Design review of the part built by this model. Coordinates are the model's own, in mm. Coordinates: 2 decimals unless noted, no trailing zeros. Write each loop counter-clockwise with the first axis right and the second up, starting at its lowest first coordinate (ties: lowest second). Pieces come first, ordered by that corner, then holes. Notation, with made-up numbers: M 32.5,-36.5 L 77.5,-36.5 A35 cw 77.5,-3.5 Z; hole C -2.75,62.5 d9. An arc over 180 degrees is marked long. Write item = value, one per line.
```python
from build123d import *

# Parameters (mm, degrees)
BOSS_EXTRUDE2_DEPTH     = 1.5875
SKETCH2_W               = 38.1
SKETCH2_H               = 76.2
BOSS_EXTRUDE3_DEPTH     = 4.7625
CUT_EXTRUDE1_DEPTH      = 1.5875
CHAMFER1_SIZE           = 2
CUT_EXTRUDE2_DEPTH      = 306.117964892
CUT_EXTRUDE2_DEPTH_BACK = 306.117964892
SKETCH4_R               = 1.25


with BuildPart() as part:
    # Sketch1 → Boss-Extrude2 (new, symmetric)
    with BuildSketch(Plane.XY.offset(250.46101)):
        with BuildLine():
            Line((-62.9, 238.2), (-40.1, 238.2))
            ThreePointArc((-40.1, 238.2), (-30.200505063, 234.099494937), (-26.1, 224.2))
            Line((-26.1, 224.2), (-26.1, -219))
            Line((-26.1, -219), (-26.1, -295.2))
            Line((-26.1, -295.2), (-76.9, -295.2))
            Line((-76.9, -295.2), (-76.9, -219))
            Line((-76.9, -219), (-76.9, 224.2))
            ThreePointArc((-76.9, 224.2), (-72.799494937, 234.099494937), (-62.9, 238.2))
        make_face()
    extrude(amount=BOSS_EXTRUDE2_DEPTH, both=True)

    # Sketch2 → Boss-Extrude3 (add, symmetric)
    with BuildSketch(Plane.XY.offset(250.46101)):
        with Locations((-51.5, -257.1)):
            Rectangle(SKETCH2_W, SKETCH2_H)
        with BuildLine():
            Line((-60.39, 231.85), (-42.61, 231.85))
            ThreePointArc((-42.61, 231.85), (-35.425795103, 228.874204897), (-32.45, 221.69))
            Line((-32.45, 221.69), (-32.45, -219))
            Line((-32.45, -219), (-70.55, -219))
            Line((-70.55, -219), (-70.55, 221.69))
            ThreePointArc((-70.55, 221.69), (-67.574204897, 228.874204897), (-60.39, 231.85))
        make_face()
    extrude(amount=BOSS_EXTRUDE3_DEPTH, both=True)

    # Sketch3 → Cut-Extrude1 (cut)
    with BuildSketch(Plane.XY.offset(255.22351)):
        with BuildLine():
            Line((-61.025, -95.175), (-61.025, -213.725))
            Line((-61.025, -213.725), (-41.975, -213.725))
            Line((-41.975, -213.725), (-41.975, -95.175))
            ThreePointArc((-41.975, -95.175), (-42.90493597, -92.92993597), (-45.15, -92))
            Line((-45.15, -92), (-57.85, -92))
            ThreePointArc((-57.85, -92), (-60.09506403, -92.92993597), (-61.025, -95.175))
        make_face()
    cut_extrude1 = extrude(amount=-CUT_EXTRUDE1_DEPTH, mode=Mode.SUBTRACT)

    # Mirror2: Cut-Extrude1 across plane
    add(cut_extrude1.mirror(Plane.XY.offset(250.46101)), mode=Mode.SUBTRACT)

    # Chamfer1
    # the kernel refuses this chamfer: 2 mm, written as the material it takes off along each edge
    with BuildSketch(Plane(origin=(-41.975, -213.725, 255.22351), x_dir=(0.999621916911297, 0, 0.0274958766105822), z_dir=(0, 1, 0))) as chamfer1_piece_1_section:
        Polygon((CHAMFER1_SIZE * 0.999621916911, CHAMFER1_SIZE * 0.0274958766106), (-CHAMFER1_SIZE * 0.0274958766106, CHAMFER1_SIZE * 0.999621916911), (0, 0), align=None)
    chamfer1_piece_1 = extrude(amount=118.55, mode=Mode.PRIVATE)
    chamfer1_piece_1 = split(chamfer1_piece_1, bisect_by=Plane(origin=(-41.282092609, -154.45, 253.63601), z_dir=(0, 0, 1)), keep=Keep.TOP, mode=Mode.PRIVATE)
    add(chamfer1_piece_1, mode=Mode.SUBTRACT)
    with BuildSketch(Plane(origin=(-61.025, -95.175, 255.22351), x_dir=(-0.999621916911297, 0, 0.0274958766105822), z_dir=(0, -1, 0))) as chamfer1_piece_2_section:
        Polygon((CHAMFER1_SIZE * 0.999621916911, CHAMFER1_SIZE * 0.0274958766106), (-CHAMFER1_SIZE * 0.0274958766106, CHAMFER1_SIZE * 0.999621916911), (0, 0), align=None)
    chamfer1_piece_2 = extrude(amount=118.55, mode=Mode.PRIVATE)
    chamfer1_piece_2 = split(chamfer1_piece_2, bisect_by=Plane(origin=(-61.717907391, -154.45, 253.63601), z_dir=(0, 0, 1)), keep=Keep.TOP, mode=Mode.PRIVATE)
    add(chamfer1_piece_2, mode=Mode.SUBTRACT)
    with BuildSketch(Plane(origin=(-45.15, -95.175, 255.22351), x_dir=(1, 0, 0), z_dir=(0, -1, 0))) as chamfer1_piece_3_section:
        Polygon((3.175 + CHAMFER1_SIZE, 0), (3.175, -CHAMFER1_SIZE), (3.175, 0), align=None)
    chamfer1_piece_3 = revolve(axis=Axis((-45.15, -95.175, 255.22351), (0, 0, 1)), revolution_arc=90, mode=Mode.PRIVATE)
    chamfer1_piece_3 = split(chamfer1_piece_3, bisect_by=Plane(origin=(-42.646845167, -92.671845167, 253.63601), z_dir=(0, 0, 1)), keep=Keep.TOP, mode=Mode.PRIVATE)
    add(chamfer1_piece_3, mode=Mode.SUBTRACT)
    with BuildSketch(Plane(origin=(-57.85, -95.175, 255.22351), x_dir=(0, 1, 0), z_dir=(1, 0, 0))) as chamfer1_piece_4_section:
        Polygon((3.175 + CHAMFER1_SIZE, 0), (3.175, -CHAMFER1_SIZE), (3.175, 0), align=None)
    chamfer1_piece_4 = revolve(axis=Axis((-57.85, -95.175, 255.22351), (0, 0, 1)), revolution_arc=90, mode=Mode.PRIVATE)
    chamfer1_piece_4 = split(chamfer1_piece_4, bisect_by=Plane(origin=(-60.353154832, -92.671845168, 253.63601), z_dir=(0, 0, 1)), keep=Keep.TOP, mode=Mode.PRIVATE)
    add(chamfer1_piece_4, mode=Mode.SUBTRACT)
    with BuildSketch(Plane(origin=(-45.15, -92, 255.22351), x_dir=(0, 0.999621916911297, 0.027495876610582105), z_dir=(-1, 0, 0))) as chamfer1_piece_5_section:
        Polygon((CHAMFER1_SIZE * 0.999621916911, CHAMFER1_SIZE * 0.0274958766106), (-CHAMFER1_SIZE * 0.0274958766106, CHAMFER1_SIZE * 0.999621916911), (0, 0), align=None)
    chamfer1_piece_5 = extrude(amount=12.7, mode=Mode.PRIVATE)
    chamfer1_piece_5 = split(chamfer1_piece_5, bisect_by=Plane(origin=(-51.5, -91.307092609, 253.63601), z_dir=(0, 0, 1)), keep=Keep.TOP, mode=Mode.PRIVATE)
    add(chamfer1_piece_5, mode=Mode.SUBTRACT)
    with BuildSketch(Plane(origin=(-41.975, -213.725, 245.69851), x_dir=(0.999621916911297, 0, -0.0274958766105822), z_dir=(0, 1, 0))) as chamfer1_piece_6_section:
        Polygon((CHAMFER1_SIZE * 0.999621916911, -CHAMFER1_SIZE * 0.0274958766106), (-CHAMFER1_SIZE * 0.0274958766106, -CHAMFER1_SIZE * 0.999621916911), (0, 0), align=None)
    chamfer1_piece_6 = extrude(amount=118.55, mode=Mode.PRIVATE)
    chamfer1_piece_6 = split(chamfer1_piece_6, bisect_by=Plane(origin=(-41.282092609, -154.45, 247.28601), z_dir=(0, 0, -1)), keep=Keep.TOP, mode=Mode.PRIVATE)
    add(chamfer1_piece_6, mode=Mode.SUBTRACT)
    with BuildSketch(Plane(origin=(-61.025, -95.175, 245.69851), x_dir=(-0.999621916911297, 0, -0.0274958766105822), z_dir=(0, -1, 0))) as chamfer1_piece_7_section:
        Polygon((CHAMFER1_SIZE * 0.999621916911, -CHAMFER1_SIZE * 0.0274958766106), (-CHAMFER1_SIZE * 0.0274958766106, -CHAMFER1_SIZE * 0.999621916911), (0, 0), align=None)
    chamfer1_piece_7 = extrude(amount=118.55, mode=Mode.PRIVATE)
    chamfer1_piece_7 = split(chamfer1_piece_7, bisect_by=Plane(origin=(-61.717907391, -154.45, 247.28601), z_dir=(0, 0, -1)), keep=Keep.TOP, mode=Mode.PRIVATE)
    add(chamfer1_piece_7, mode=Mode.SUBTRACT)
    with BuildSketch(Plane(origin=(-45.15, -95.175, 245.69851), x_dir=(1, 0, 0), z_dir=(0, -1, 0))) as chamfer1_piece_8_section:
        Polygon((3.175 + CHAMFER1_SIZE, 0), (3.175, CHAMFER1_SIZE), (3.175, 0), align=None)
    chamfer1_piece_8 = revolve(axis=Axis((-45.15, -95.175, 245.69851), (0, 0, 1)), revolution_arc=90, mode=Mode.PRIVATE)
    chamfer1_piece_8 = split(chamfer1_piece_8, bisect_by=Plane(origin=(-42.646845167, -92.671845167, 247.28601), z_dir=(0, 0, -1)), keep=Keep.TOP, mode=Mode.PRIVATE)
    add(chamfer1_piece_8, mode=Mode.SUBTRACT)
    with BuildSketch(Plane(origin=(-57.85, -95.175, 245.69851), x_dir=(0, 1, 0), z_dir=(1, 0, 0))) as chamfer1_piece_9_section:
        Polygon((3.175 + CHAMFER1_SIZE, 0), (3.175, CHAMFER1_SIZE), (3.175, 0), align=None)
    chamfer1_piece_9 = revolve(axis=Axis((-57.85, -95.175, 245.69851), (0, 0, 1)), revolution_arc=90, mode=Mode.PRIVATE)
    chamfer1_piece_9 = split(chamfer1_piece_9, bisect_by=Plane(origin=(-60.353154832, -92.671845168, 247.28601), z_dir=(0, 0, -1)), keep=Keep.TOP, mode=Mode.PRIVATE)
    add(chamfer1_piece_9, mode=Mode.SUBTRACT)
    with BuildSketch(Plane(origin=(-45.15, -92, 245.69851), x_dir=(0, 0.999621916911297, -0.027495876610582105), z_dir=(-1, 0, 0))) as chamfer1_piece_10_section:
        Polygon((CHAMFER1_SIZE * 0.999621916911, -CHAMFER1_SIZE * 0.0274958766106), (-CHAMFER1_SIZE * 0.0274958766106, -CHAMFER1_SIZE * 0.999621916911), (0, 0), align=None)
    chamfer1_piece_10 = extrude(amount=12.7, mode=Mode.PRIVATE)
    chamfer1_piece_10 = split(chamfer1_piece_10, bisect_by=Plane(origin=(-51.5, -91.307092609, 247.28601), z_dir=(0, 0, -1)), keep=Keep.TOP, mode=Mode.PRIVATE)
    add(chamfer1_piece_10, mode=Mode.SUBTRACT)

    # Sketch4 → Cut-Extrude2 (cut, two sides: drawn at the far end of the back side and taken through both)
    with BuildSketch(Plane.XY.offset(252.04851).offset(-CUT_EXTRUDE2_DEPTH_BACK)):
        with Locations((-61.025, -231.7)):
            Circle(SKETCH4_R)
        with Locations((-41.975, -231.7)):
            Circle(SKETCH4_R)
        with Locations((-35.625, -282.5)):
            Circle(SKETCH4_R)
        with Locations((-67.375, -282.5)):
            Circle(SKETCH4_R)
    extrude(amount=CUT_EXTRUDE2_DEPTH + CUT_EXTRUDE2_DEPTH_BACK, mode=Mode.SUBTRACT)


solid = part.part
```
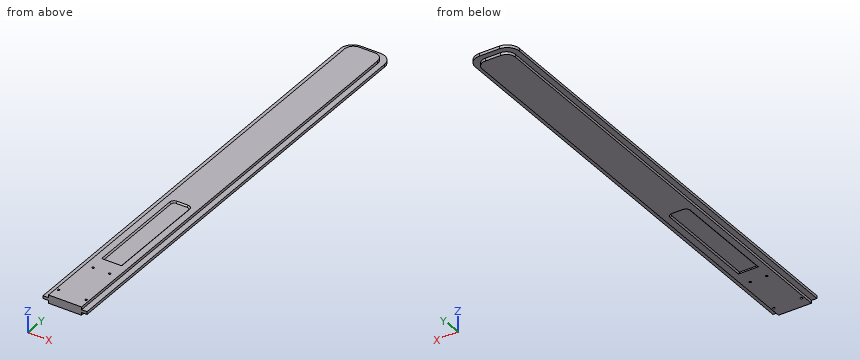
Q1. Wall thickness on line 1 (X direction, y = -282.5, z = 251) (3 decimals); line 2 (X direction, y = -231.7, z = 251.5) (3 decimals); line 3 (X direction, y = 104.5, z = 254.5): over which ranges is each line inside the solid? List them lowest first.
Check result:
line_1 = -76.9 to -68.625, -66.125 to -36.875, -34.375 to -26.1
line_2 = -76.9 to -62.275, -59.775 to -43.225, -40.725 to -26.1
line_3 = -70.55 to -32.45
Q2. Consider section A-A, the plane y = -245.5. State the section outline as (x, z) points, and give its area (3 significant figures).
Check result:
outline = M -76.9,248.87 L -70.55,248.87 L -70.55,245.7 L -32.45,245.7 L -32.45,248.87 L -26.1,248.87 L -26.1,252.05 L -32.45,252.05 L -32.45,255.22 L -70.55,255.22 L -70.55,252.05 L -76.9,252.05 Z
area = 403 mm²
Q3. For P1, Ø2, axis at x = -67.375, y = -282.5, coming from the -Z side; P2, Ø1.6, axis at y = 89.5, z = 247.5, coming from the -X side; P3, Ø0.5, axis at x = -54, z = 254, coming from the +Y side; P4, Ø16, axis at x = -53, y = -157, coming from the -Z side, all flat-tipped, find the tip position at first contact; note any pin that passes through.
Check result:
P1 = through
P2 = -70.55
P3 = 231.85
P4 = 247.29
